from build123d import *

# Parameters (mm, degrees)
SKETCH_1_W          = 21
SKETCH_1_H          = 34
EXTRUDE_1_DEPTH     = 9
SKETCH_6_W          = 13.003696042
SKETCH_6_H          = 17
CUT_EXTRUDE_3_DEPTH = 22.914607001
CUT_EXTRUDE_4_DEPTH = 1.8
CUT_EXTRUDE_5_REACH = 29.178
SKETCH_11_R         = 1.65
CUT_EXTRUDE_6_DEPTH = 3
CUT_EXTRUDE_7_REACH = 22.863
SKETCH_16_R         = 1.2
CUT_EXTRUDE_8_DEPTH = 1.8


with BuildPart() as part:
    # 草图1 → 凸台-拉伸1 (new body)
    with BuildSketch(Plane(origin=(0, 0, 0), x_dir=(1, 0, 0), z_dir=(0, 1, 0))):
        Rectangle(SKETCH_1_W, SKETCH_1_H)
    extrude(amount=EXTRUDE_1_DEPTH)

    # 草图6 → 切除-拉伸3 (cut, through all)
    with BuildSketch(Plane(origin=(0, 9, 0), x_dir=(1, 0, 0), z_dir=(0, 1, 0))):
        with Locations((0, -8.5)):
            Rectangle(SKETCH_6_W, SKETCH_6_H)
    extrude(amount=-CUT_EXTRUDE_3_DEPTH, mode=Mode.SUBTRACT)

    # 草图9 → M3 六角圆柱头螺钉的柱形沉头孔1 (revolve, cut)
    with BuildSketch(Plane(origin=(10.5, 4.5, 11.5), x_dir=(0, 0, -1), z_dir=(0, 1, 0))):
        Polygon((0, 0), (0, 3.998151979), (1.7, 3.998151979), (1.7, 3.4), (3, 3.4), (3, 0.025), (3.025, 0), align=None)
    revolve(axis=Axis((16.85, 4.5, 11.5), (-1, 0, 0)), mode=Mode.SUBTRACT)

    # 草图10 → 切除-拉伸4 (cut)
    with BuildSketch(Plane.ZY.offset(10.5)):
        Polygon((13.174315781, 1.6), (14.848631561, 4.5), (13.174315781, 7.4), (9.825684219, 7.4), (8.151368439, 4.5), (9.825684219, 1.6), align=None)
    extrude(amount=-CUT_EXTRUDE_4_DEPTH, mode=Mode.SUBTRACT)

    # 草图11 → 切除-拉伸5 (cut, up to next)
    with BuildSketch(Plane.ZY.offset(8.7), mode=Mode.PRIVATE) as cut_extrude_5_sk1:
        with Locations((11.5, 4.5)):
            Circle(SKETCH_11_R)
    cut_extrude_5_tool1 = extrude(cut_extrude_5_sk1.sketch, amount=-CUT_EXTRUDE_5_REACH, mode=Mode.PRIVATE) & part.part
    add(cut_extrude_5_tool1.solids().sort_by_distance((-8.7, 4.5, 11.5))[0], mode=Mode.SUBTRACT)

    # 草图12 → 切除-拉伸6 (cut)
    with BuildSketch(Plane(origin=(0, 3, 0), x_dir=(-1, 0, 0), z_dir=(0, -1, 0))):
        with BuildLine():
            Line((-10.5, 17), (10.5, 17))
            Line((10.5, 17), (10.5, 3.552777817))
            ThreePointArc((10.5, 3.552777817), (0, 3), (-10.5, 3.552777817))
            Line((-10.5, 3.552777817), (-10.5, 17))
        make_face()
    extrude(amount=-CUT_EXTRUDE_6_DEPTH, mode=Mode.SUBTRACT)

    # 草图15 → M2 六角圆柱头螺钉的柱形沉头孔1 (revolve, cut)
    with BuildSketch(Plane(origin=(0, 9, -8), x_dir=(0, 0, 1), z_dir=(1, 0, 0))):
        Polygon((0, 0), (0, 3), (1.2, 3), (1.2, 2.3), (2.15, 2.3), (2.15, 0.025), (2.175, 0), align=None)
    revolve(axis=Axis((0, 15.35, -8), (0, -1, 0)), mode=Mode.SUBTRACT)

    # 草图16 → 切除-拉伸7 (cut, up to next)
    with BuildSketch(Plane(origin=(0, 3, 0), x_dir=(1, 0, 0), z_dir=(0, 1, 0)), mode=Mode.PRIVATE) as cut_extrude_7_sk1:
        with Locations(Location((0, 8, 0), (0, 0, 270))):
            Circle(SKETCH_16_R)
    cut_extrude_7_tool1 = extrude(cut_extrude_7_sk1.sketch, amount=-CUT_EXTRUDE_7_REACH, mode=Mode.PRIVATE) & part.part
    add(cut_extrude_7_tool1.solids().sort_by_distance((0, 3, -8))[0], mode=Mode.SUBTRACT)

    # 草图17 → 切除-拉伸8 (cut)
    with BuildSketch(Plane.XZ):
        Polygon((1.212435565, -10.1), (2.424871131, -8), (1.212435565, -5.9), (-1.212435565, -5.9), (-2.424871131, -8), (-1.212435565, -10.1), align=None)
    extrude(amount=-CUT_EXTRUDE_8_DEPTH, mode=Mode.SUBTRACT)


solid = part.part
Read the model definition and answer for the solid it produces. Units are mm, in the model's axes. A direction names the side the tool comes from. Coordinates: 2 decimals unless noted, no trailing zeros. Write each loop counter-clockwise with the first axis right and the second up, starting at its lowest first coordinate (ties: lowest second). Pieces come first, ordered by that corner, then holes. Notation, with made-up numbers: M 85.5,-30.75 L 117.5,-30.75 A19 ccw 117.5,-18.75 Z; hole C 38,-35.75 d2. An arc over 180 degrees is marked long. Use a Markdown table: item, result.
Q1. Each of these flat-tipped pins is pushed along its axis until it touches: pin 1 Ø4.5 at (x, y) = (0.5, 5.5) entering from +Z; pin 2 Ø3 at (y, z) = (3.5, 12) entering from +X; pin 3 Ø1.4 at (x, z) = (0, -8) entering from -Y; pin 4 Ø1.7 at (y, z) = (3.5, 11.5) entering from -X. Where does it stop, or does it pass through?
Answer block:
| item | result |
|---|---|
| pin 1 | stops at z = 0 |
| pin 2 | stops at x = 7.1 |
| pin 3 | passes through |
| pin 4 | stops at x = -8.7 |
Q2. The part is cut by section D-D, the plane y = 1. Write down the section's boundary in (x, z), then the cut area to 3 significant figures.
Answer block:
| item | result |
|---|---|
| outline | M -10.5,-17 L 10.5,-17 L 10.5,17 L 6.5,17 L 6.5,0 L -6.5,0 L -6.5,17 L -10.5,17 Z; hole M -2.42,-8 L -1.21,-10.1 L 1.21,-10.1 L 2.42,-8 L 1.21,-5.9 L -1.21,-5.9 Z |
| area | 478 mm2 |
Q3. The part is cut by section A-A, the plane z = -14. Write down the section's boundary in (x, y).
Answer block:
| item | result |
|---|---|
| outline | M -10.5,0 L 10.5,0 L 10.5,3 L -10.5,3 Z; M -10.5,6 L 10.5,6 L 10.5,9 L -10.5,9 Z |
Q4. Which of the six approach directions +Z, -Z, +X, -X, +Y, -Y give full straight-line access (tool end or side, diameter ignored) to faces 4 (the face through (-1.827, 0.887, -9.035)), 5 (the face through (8.81, 2.47, 13.71)), 6 (the face through (-9.61, 3.03, 14)), 7 (the face through (6.502, 5, 9)), 8 (the face through (0, 1, -17))?
Answer block:
| item | result |
|---|---|
| face 4 | -Y |
| face 5 | +X |
| face 6 | -X |
| face 7 | +Z, +Y, -Y |
| face 8 | -Z, +X, -X, +Y, -Y |
Q5. The part is cut by section B-B, the plane x = 0. Write down the section's boundary in (y, z) (3 decimals).
Answer block:
| item | result |
|---|---|
| outline | M 0,-17 L 3,-17 L 3,-9.2 L 1.8,-9.2 L 1.8,-10.1 L 0,-10.1 Z; M 0,-5.9 L 1.8,-5.9 L 1.8,-6.8 L 3,-6.8 L 3,-3 L 6,-3 L 6,-6.8 L 6.7,-6.8 L 6.7,-5.85 L 8.975,-5.85 L 9,-5.825 L 9,0 L 0,0 Z; M 6,-17 L 9,-17 L 9,-10.175 L 8.975,-10.15 L 6.7,-10.15 L 6.7,-9.2 L 6,-9.2 Z |
Q6. Determine the mould class of faces 1 (the face through (8, 4, 17)), 2 (the face through (6.81, 5.15, 9.93)), 3 (the face through (0, 0, -4)) for opening direction Y: released by +Y, released by -Y, zero draft, split by the parting line, or undercut.
Answer block:
| item | result |
|---|---|
| face 1 | zero draft |
| face 2 | undercut |
| face 3 | released by -Y |
Q7. Straight lines are drawn through the part: L1, parallel to X at y = 2.75, z = -8; L2, parallel to X at y = 1.75, z = 13.5; L3, parallel to Y at x = -7.8, z = 11.5. For each, find the intervals that lie inside material, in ascending order. Write a range as [from, to].
Answer block:
| item | result |
|---|---|
| L1 | x = [-10.5, -1.2], [1.2, 10.5] |
| L2 | x = [-10.5, -6.5], [6.5, 10.5] |
| L3 | y = [0, 2.85], [6.15, 9] |
Q8. The part is cut by section C-C, the plane z = 11.5. Write down the section's boundary in (x, y) (3 decimals), then the cut area to 3 significant figures.
Answer block:
| item | result |
|---|---|
| outline | M -10.5,0 L -6.502,0 L -6.502,2.85 L -8.7,2.85 L -8.7,1.6 L -10.5,1.6 Z; M -10.5,7.4 L -8.7,7.4 L -8.7,6.15 L -6.502,6.15 L -6.502,9 L -10.5,9 Z; M 6.502,0 L 10.5,0 L 10.5,1.475 L 10.475,1.5 L 7.1,1.5 L 7.1,2.8 L 6.502,2.8 Z; M 6.502,6.2 L 7.1,6.2 L 7.1,7.5 L 10.475,7.5 L 10.5,7.525 L 10.5,9 L 6.502,9 Z |
| area | 31.8 mm2 |
